Work out the finished part from the listing and answer in its coordinate system (mm). A direction names the side the tool comes from. Coordinates: 2 decimals unless noted, no trailing zeros. Write each loop counter-clockwise with the first axis right and the second up, starting at its lowest first coordinate (ties: lowest second). Pieces come first, ordered by that corner, then holes. Notation, with made-up numbers: (85.5, 81) - (109.5, 81) arc R28 cw to (109.5, 105) - close; hole circle Ø8 at (64, -28.5). An arc over 180 degrees is marked (long way). Use a Markdown table: item, result. Add a question column.
(1) The part is cut by section A-A, the plane x = 0. Give the vertices of the cut face in (y, z), then the cut area to 3 significant figures.
(2) The part is cut by section B-B, the plane y = 2. Give the vertices of the cut face in (x, z), then the cut area to 3 significant figures.
(3) Given pin 1 Ø3 at (y, z) = (-14, 0.5) entering from +X; pin 2 Ø1 at (y, z) = (12, 0) entering from +X; pin 3 Ø1.5 at (x, z) = (7, 2) entering from -Y, each flat-ended and moving along its own axis, determine where each tip first touches the part or whether it passes through.
(4) A tool of negligible diameter and unlimited length cuts with its end or side. For faces 5 (the face through (-4.78, 14.13, 0.06)), 6 (the face through (0.07, 26.394, -0.063)), from which of +Z, -Z, +X, -X, +Y, -Y can it reach the whole face along a straight path? Write none if from no direction.
(5) Find the intervals of material crossed by line 1 (X direction, y = -6, z = -3.5); line 2 (X direction, y = 14.5, z = -1.5); line 3 (Y direction, x = 1, z = -3.5), in increasing order. Write a range as from..to.
(6) For a pull along X with two mould halves and no side action, classify faces 1 (the face through (-17.504, 0.181, 0.063)), 2 (the face through (0.07, -26.394, -0.063)), 3 (the face through (-7.504, 0.153, 0.063)), 4 (the face through (-8, 0, 4.5)) as released by +X, released by -X, zero draft, split by the parting line, or undercut.
from build123d import *

# Parameters (mm, degrees)
F1_DEPTH    = 4.5
F2_R        = 17
F3_T1_DEPTH = 33.9045095963
F5_DEPTH    = 9


# Not quite as in the source:
# - a fillet or chamfer that OpenCascade refuses, or shapes differently, is made with other operations: its cross-section is extruded or revolved along the edge and cut away or added


with BuildPart() as f1:
    # F0 (on Top) → F1 (new body, symmetric)
    with BuildSketch(Plane.XY):
        with BuildLine():
            ThreePointArc((15.375, -16.5), (17.5041005313, 0), (15.375, 16.5))
            ThreePointArc((15.375, 16.5), (9.0566864996, 23.6051242432), (0, 26.5))
            ThreePointArc((0, 26.5), (-9.0566864996, 23.6051242432), (-15.375, 16.5))
            ThreePointArc((-15.375, 16.5), (-17.5041005313, 0), (-15.375, -16.5))
            ThreePointArc((-15.375, -16.5), (-9.0566864996, -23.6051242432), (0, -26.5))
            ThreePointArc((0, -26.5), (9.0566864996, -23.6051242432), (15.375, -16.5))
        make_face()
    extrude(amount=F1_DEPTH, both=True)

    # F2
    f2_edges = [f1.edges().sort_by_distance(p)[0] for p in [
        (-15.375, 16.5, 0),
        (-15.375, -16.5, 0),
        (15.375, -16.5, 0),
        (15.375, 16.5, 0),
    ]]
    fillet(f2_edges, radius=F2_R)

    # F3: fillet of radius 15.59 on 2 edges, made by hand

    # F3_s2 → F3_t1 (cut)
    with BuildSketch(Plane.XY.offset(-16.9522547982)):
        with BuildLine():
            ThreePointArc((4.8996291219, 25.603887062), (0, 26.3938284652), (-4.8996291219, 25.603887062))
            ThreePointArc((-4.8996291219, 25.603887062), (-2.4809605234, 26.222238656), (0, 26.5))
            ThreePointArc((0, 26.5), (2.4809605234, 26.222238656), (4.8996291219, 25.603887062))
        make_face()
        with BuildLine():
            ThreePointArc((4.8996291219, -25.603887062), (0, -26.3938284652), (-4.8996291219, -25.603887062))
            ThreePointArc((-4.8996291219, -25.603887062), (-2.4809605234, -26.222238656), (0, -26.5))
            ThreePointArc((0, -26.5), (2.4809605234, -26.222238656), (4.8996291219, -25.603887062))
        make_face()
    extrude(amount=F3_T1_DEPTH, mode=Mode.SUBTRACT)

    # F4 (on face) → F5 (cut, through all)
    with BuildSketch(Plane.XY.offset(4.5)):
        with BuildLine():
            ThreePointArc((-6.424547387, 10.8436806891), (-7.5041005313, 0), (-6.424547387, -10.8436806891))
            ThreePointArc((-6.424547387, -10.8436806891), (-4.8148810997, -14.0903093829), (-1.797468323, -16.0970090531))
            ThreePointArc((-1.797468323, -16.0970090531), (-1.7771565537, -16.1038240182), (-1.7568266062, -16.1105845625))
            ThreePointArc((-1.7568266062, -16.1105845625), (0, -16.3938284652), (1.7568266062, -16.1105845625))
            ThreePointArc((1.7568266062, -16.1105845625), (1.7771565537, -16.1038240182), (1.797468323, -16.0970090531))
            ThreePointArc((1.797468323, -16.0970090531), (4.8148810997, -14.0903093829), (6.424547387, -10.8436806891))
            ThreePointArc((6.424547387, -10.8436806891), (7.5041005313, 0), (6.424547387, 10.8436806891))
            ThreePointArc((6.424547387, 10.8436806891), (4.8148810997, 14.0903093829), (1.797468323, 16.0970090531))
            ThreePointArc((1.797468323, 16.0970090531), (1.7771565537, 16.1038240182), (1.7568266062, 16.1105845625))
            ThreePointArc((1.7568266062, 16.1105845625), (0, 16.3938284652), (-1.7568266062, 16.1105845625))
            ThreePointArc((-1.7568266062, 16.1105845625), (-1.7771565537, 16.1038240182), (-1.797468323, 16.0970090531))
            ThreePointArc((-1.797468323, 16.0970090531), (-4.8148810997, 14.0903093829), (-6.424547387, 10.8436806891))
        make_face()
    extrude(amount=-F5_DEPTH, mode=Mode.SUBTRACT)


solid = f1.part
Model answer:
| question | item | result |
|---|---|---|
| 1 | outline | (-26.39, -4.5) - (-16.39, -4.5) - (-16.39, 4.5) - (-26.39, 4.5) - close; (16.39, -4.5) - (26.39, -4.5) - (26.39, 4.5) - (16.39, 4.5) - close |
| 1 | area | 180 mm^2 |
| 2 | outline | (-17.47, -4.5) - (-7.47, -4.5) - (-7.47, 4.5) - (-17.47, 4.5) - close; (7.47, -4.5) - (17.47, -4.5) - (17.47, 4.5) - (7.47, 4.5) - close |
| 2 | area | 180 mm^2 |
| 3 | pin 1 | x = 16.29 |
| 3 | pin 2 | x = 16.48 |
| 3 | pin 3 | y = -25.09 |
| 4 | face 5 | +Z, -Z |
| 4 | face 6 | +Z, -Z, +Y |
| 5 | line 1 | -17.23..-7.18, 7.18..17.23 |
| 5 | line 2 | -15.8..-4.42, 4.42..15.8 |
| 5 | line 3 | -26.36..-16.3, 16.3..26.36 |
| 6 | face 1 | released by -X |
| 6 | face 2 | split by the parting line |
| 6 | face 3 | undercut |
| 6 | face 4 | zero draft |
